Autodesk Inventor part; units mm, degrees
ref_plane "YZ Plane" through (0, 0, 0) normal (1, 0, 0) x (0, 1, 0)
ref_plane "XZ Plane" through (0, 0, 0) normal (0, 1, 0) x (-1, 0, 0)
ref_plane "XY Plane" through (0, 0, 0) normal (0, 0, 1) x (1, 0, 0)
sketch "Sketch1" plane through (0, 0, 0) normal (0, 1, 0) x (-1, 0, 0)
  circle A0 centre (0, 0) radius 26
  dimension "d0" = 52
extrude "Extrusion1" add sketch "Sketch1" along normal blind 12
sketch "Sketch2" plane through (0, 12, 0) normal (0, 1, 0) x (1, 0, 0)
  circle A0 centre (0, 0) radius 16
  dimension "d3" = 32
extrude "Extrusion2" cut sketch "Sketch2" against normal blind 10
sketch "Sketch3" plane through (0, 2, 0) normal (0, 1, 0) x (1, 0, 0)
  circle A0 centre (0, 0) radius 12
  dimension "d6" = 24
extrude "Extrusion3" cut sketch "Sketch3" against normal through all
sketch "Sketch4" plane through (0, 0, 0) normal (0, -1, 0) x (1, 0, 0)
  circle A0 centre (0, 0) radius 14
  circle A1 centre (0, 0) radius 12
  dimension "d9" = 2
extrude "Extrusion4" add sketch "Sketch4" along normal blind 2
sketch "Sketch5" plane through (0, 0, 0) normal (0, -1, 0) x (1, 0, 0)
  circle A0 centre (0, 0) radius 16
  circle A1 centre (0, 0) radius 16
  circle A2 centre (0, 0) radius 26
  circle A3 centre (0, 0) radius 21 construction
  line L0 (0, 36.4) -> (0, -36.4) construction
  point P0 (0, 21)
  point P1 (-18.1865, -10.5)
  point P2 (18.1865, -10.5)
  dimension "d12" = 5
  dimension "d15" = 360
hole "Hole1" at (0, 0, 21) at (-18.1865, 0, -10.5) at (18.1865, 0, -10.5) direction (0, 1, 0) diameter 2.459 end through all
chamfer "Chamfer1" distance 0.5 angle 60 3 edges at (0, 0, 22.2295) (-18.1865, 0, -9.2705) (18.1865, 0, -9.2705) measured on face at (-13.3646, 0, -14.7799)
chamfer "Chamfer2" distance 0.3 angle 45 1 edges at (-14, -2, 0)
properties part number "ball bearing mount"
Check sheet for the modelled part. Datum: model origin and axes. Units: mm. A direction names the side the tool comes from. Give positions to 0.01 mm unless a question says otherwise; leave off trailing zeros. Order: outer loops, then holes, each group sorted by start corner. A loop starts at its lowest first (then second) coordinate and runs counter-clockwise, first axis right, second up. Notation, with made-up numbers: (-29.5, 30) -> (-2.5, 30) arc R24 cw to (-2.5, 60) -> close; hole circle Ø11 at (69, -26). An arc over 180 degrees is marked (long way). Use CSV: the item, a comma, the result in double quotes. Start each with the question number.
1) Sectioned sample at D-D, the plane y = 6.5. Record the boundary of the cut face in (x, z), plus the area to 3 significant figures.
2) Go/stop test with flat-tipped pins: P1, Ø8, axis at x = 18, y = 0.5, coming from the +Z side; P2, Ø2, axis at y = 0.5, z = -17, coming from the -X side; P3, Ø4, axis at x = -2.5, y = 9, coming from the +Z side. Record where each tip stops, or that it passes through.
3) Set-up check for faces 1 (the face through (-11, 0, -11)), 2 (the face through (-3.47, 7.07, 15.62)), 3 (the face through (0.951, -2, -12.114)): record each of +Z, -Z, +X, -X, +Y, -Y from which the full face is reachable in a straight line by a thin tool's end or side.
4) Sectioned sample at C-C, the plane z = 21. Record the boundary of the cut face in (x, y), plus the area to 3 significant figures.
5) Mould release check, pull along X, two halves, no side actions. Record for faces 4 (the face through (2, 2, -12)), 5 (the face through (-11, 12, 12)), 6 (the face through (20.633, 5.916, 15.821)): released by +X, released by -X, zero draft, split by the parting line, or undercut.
6) Material ranges on line 1 (Z direction, x = 0, y = 5); line 2 (Y direction, x = -9.5, z = -20); line 3 (X direction, y = 8, z = 21.5), recorded low to high. Write a range as from..to.
7) Sectioned sample at B-B, the plane x = 0. Record the boundary of the cut face in (y, z), plus the area to 3 significant figures.
8) Sectioned sample at A-A, the plane z = 0. Record the boundary of the cut face in (x, y), plus the area to 3 significant figures.
Recorded:
1,outline,"circle Ø52 at (0, 0); hole circle Ø2.46 at (-18.19, -10.5); hole circle Ø32 at (0, 0); hole circle Ø2.46 at (0, 21); hole circle Ø2.46 at (18.19, -10.5)"
1,area,"1,310 mm2"
2,P1,"z = 21.91"
2,P2,"x = -20.49"
2,P3,"z = 26"
3,face 1,"-Y"
3,face 2,"+Y"
3,face 3,"+Z, -Z, +X, -X, -Y"
4,outline,"(-15.33, 0) -> (-1.73, 0) -> (-1.23, 0.87) -> (-1.23, 12) -> (-15.33, 12) -> close; (1.23, 0.87) -> (1.73, 0) -> (15.33, 0) -> (15.33, 12) -> (1.23, 12) -> close"
4,area,"338 mm2"
5,face 4,"undercut"
5,face 5,"zero draft"
5,face 6,"split by the parting line"
6,line 1,"-26..-16, 16..19.77, 22.23..26"
6,line 2,"0..12"
6,line 3,"-14.62..-1.12, 1.12..14.62"
7,outline,"(-2, -13.7) -> (-1.7, -14) -> (0, -14) -> (0, -26) -> (12, -26) -> (12, -16) -> (2, -16) -> (2, -12) -> (-2, -12) -> close; (-2, 12) -> (2, 12) -> (2, 16) -> (12, 16) -> (12, 19.77) -> (0.87, 19.77) -> (0, 19.27) -> (0, 14) -> (-1.7, 14) -> (-2, 13.7) -> close; (0, 22.73) -> (0.87, 22.23) -> (12, 22.23) -> (12, 26) -> (0, 26) -> close"
7,area,"234 mm2"
8,outline,"(-26, 0) -> (-14, 0) -> (-14, -1.7) -> (-13.7, -2) -> (-12, -2) -> (-12, 2) -> (-16, 2) -> (-16, 12) -> (-26, 12) -> close; (12, -2) -> (13.7, -2) -> (14, -1.7) -> (14, 0) -> (26, 0) -> (26, 12) -> (16, 12) -> (16, 2) -> (12, 2) -> close"
8,area,"264 mm2"
